Geometry: see drawing. Coordinates: mm, zero at the bounding-box minimum. Round coordinates to 2 decimals unless told otherwise and drop trailing zeros. Loops run counter-clockwise (first coordinate to the right, second up) from the corner with the lowest first, then second, coordinate; pieces in that order, holes last.
(1) Cut plane C-C, the plane y = 7.25. Output: boundary loops of the cut face in (x, z).
(2) Cut plane A-A, the plane x = 2.5. Output: boundary loops of the cut face in (y, z), and give its area (3 significant figures).
(3) Draft query along X for the marked faces 1, 2 and 3. Return one class per face: released by +X, released by -X, zero draft, split by the parting line, or undercut.
(4) First-contact query: pin 1 Ø1.7 at (x, y) = (2.5, 6.5) entering from -Z. Flat tip, straight axial feed; report the tip coordinate or a pass-through.
(5) Cut plane D-D, the plane z = 5.25. Output: boundary loops of the cut face in (x, y).
(6) Cut plane B-B, the plane z = 1.75. Output: boundary loops of the cut face in (x, y), and give its area (3 significant figures).
(7) Line query: line 1 (Y direction, x = 2.5, z = 2.25); line 2 (X direction, y = 6.5, z = 2.75); line 3 (X direction, y = 7, z = 3.25). Output: solid intervals per line, ascending.
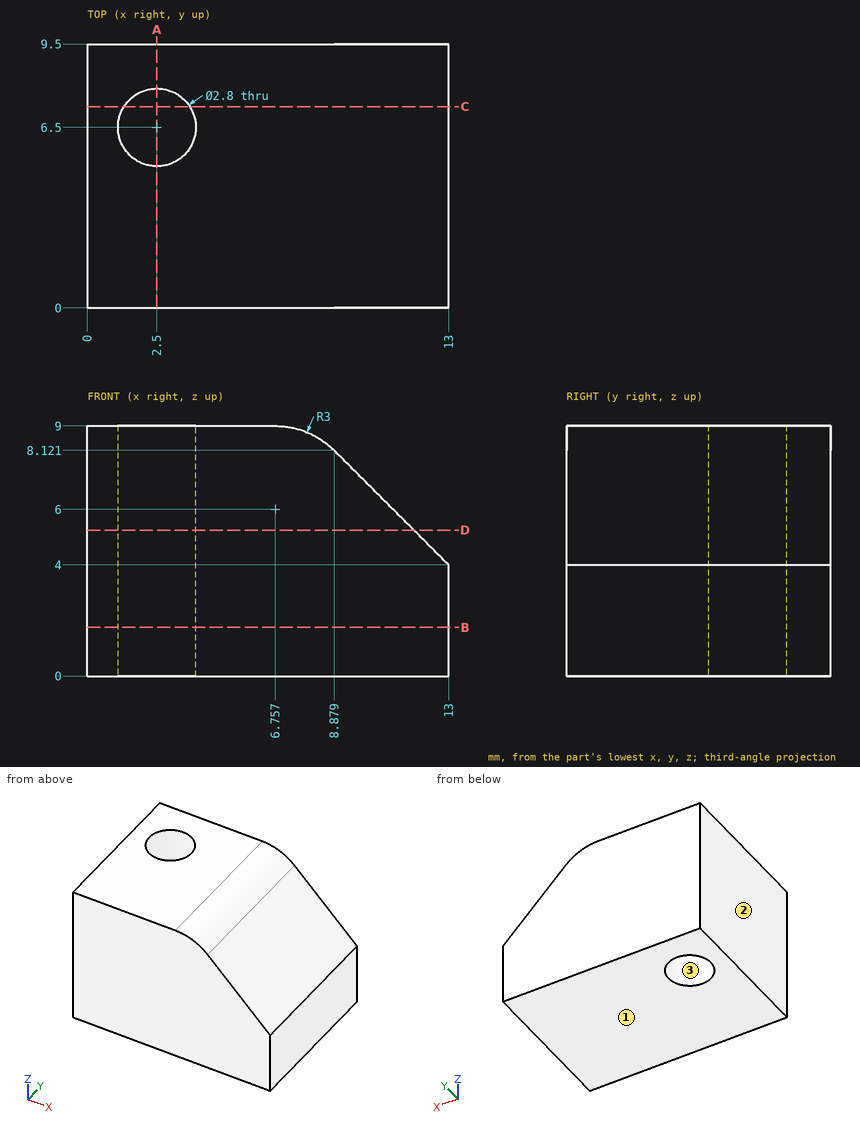
Reported:
1. outline: (0, 0) - (1.32, 0) - (1.32, 9) - (0, 9) - close; (3.68, 0) - (13, 0) - (13, 4) - (8.88, 8.12) arc R3 ccw to (6.76, 9) - (3.68, 9) - close
2. outline: (0, 0) - (5.1, 0) - (5.1, 9) - (0, 9) - close; (7.9, 0) - (9.5, 0) - (9.5, 9) - (7.9, 9) - close
2. area: 60.3 mm2
3. face 1: zero draft
3. face 2: released by -X
3. face 3: undercut
4. pin 1: passes through
5. outline: (0, 0) - (11.75, 0) - (11.75, 9.5) - (0, 9.5) - close; hole circle Ø2.8 at (2.5, 6.5)
6. outline: (0, 0) - (13, 0) - (13, 9.5) - (0, 9.5) - close; hole circle Ø2.8 at (2.5, 6.5)
6. area: 117 mm2
7. line 1: y = 0 to 5.1, 7.9 to 9.5
7. line 2: x = 0 to 1.1, 3.9 to 13
7. line 3: x = 0 to 1.19, 3.81 to 13
